Geometry check sheet. Reference: the model listing, model coordinates, mm. A direction names the side the tool comes from. Round coordinates to 2 decimals unless told otherwise and drop trailing zeros. Write each loop counter-clockwise with the first axis right and the second up, starting at its lowest first coordinate (ties: lowest second). Pieces come first, ordered by that corner, then holes. Notation, with made-up numbers: M 28,17 L 84,17 A15 cw 84,29 Z; hole C -5.75,59.5 d11. An arc over 180 degrees is marked long. Answer in a Markdown table with one row per item. Add a question column.
Autodesk Inventor part; units mm, degrees
ref_plane "YZ Plane" through (0, 0, 0) normal (1, 0, 0) x (0, 1, 0)
ref_plane "XZ Plane" through (0, 0, 0) normal (0, 1, 0) x (-1, 0, 0)
ref_plane "XY Plane" through (0, 0, 0) normal (0, 0, 1) x (1, 0, 0)
sketch "Sketch1" plane through (0, 0, 0) normal (0, 0, 1) x (1, 0, 0)
  line L0 (0, 0) -> (-18, 0)
  line L1 (-18, 0) -> (-19.55, 1.55)
  line L2 (-19.55, 1.55) -> (-19.55, 4.95)
  line L3 (-19.55, 4.95) -> (-18, 6.5)
  line L4 (-18, 6.5) -> (-14.45, 6.5)
  line L5 (-14.45, 6.5) -> (-14.45, 3.05)
  line L6 (-14.45, 3.05) -> (0, 3.05)
  line L7 (0, 3.05) -> (0, 0)
  point P0 (-19.55, 3.25)
  dimension "d0" = 3.05
  dimension "d1" = 14.45
  dimension "d2" = 6.5
  dimension "d3" = 5.1
  dimension "d4" = 3.4
  dimension "d5" = 3.25
  dimension "d6" = 3.55
extrude "Extrusion1" add sketch "Sketch1" along normal blind 0.55
ref_plane "Work Plane1" through (-14.45, 1.525, 0) normal (0, 1, 0) x (1, 0, 0)
sketch "Sketch2" plane through (-14.45, 1.525, 0) normal (0, 1, 0) x (1, 0, 0)
  line L0 (14.45, -0.55) -> (0, -0.55)
  line L1 (14.45, 0) -> (14.45, -0.55)
  line L2 (7.75, -0.55) -> (11.15, -0.55)
  line L3 (11.15, -0.55) -> (11.15, -2.25)
  line L4 (11.15, -2.25) -> (7.75, -2.25)
  line L5 (7.75, -2.25) -> (7.75, -0.55)
  line L6 (11.15, -0.55) -> (12.475, -1.875)
  line L7 (12.475, -1.875) -> (12.275, -0.55)
  line L8 (7.75, -0.55) -> (6.425, -1.875)
  line L9 (6.425, -1.875) -> (6.625, -0.55)
  line L10 (6.625, -0.55) -> (7.75, -0.55)
  line L11 (11.15, -0.55) -> (12.275, -0.55)
  point P0 (9.45, -2.25)
  dimension "d9" = 3.3
  dimension "d10" = 3.4
  dimension "d11" = 1.7
  dimension "d14" = 6.05
  dimension "d15" = 3.025
  dimension "d16" = 5.65
extrude "Extrusion2" add sketch "Sketch2" along normal mid plane 0.5
fillet "Fillet1" radius 0.2 2 edges at (-8.025, 1.525, 1.875) (-1.975, 1.525, 1.875)
properties part number "Soanar Power Module Pin E" material "Nickel-Copper Alloy 400"
Item 1: Section check D-D, the plane z = 1.8. Record the boundary of the cut face in (x, y) (3 decimals), and give its area (3 significant figures).
Item 2: Mould release check, pull along X, two halves, no side actions. Record for faces 1 (the flat face through (-2.86, 1.52, 0.99)), 2 (the flat face through (-18.8, 0.8, 0.3)), 3 (the flat face through (-2.6, 1.275, 0.9)): +X half, -X half, draft (parallel to the pull), parting line (faces both ways), or undercut.
Item 3: Section check A-A, the plane x = -6. Record the boundary of the cut face in (y, z) (3 decimals).
Item 4: Gauge pin test, flat ends, axial feed: pin 1 Ø0.5 at (x, z) = (-7, 1) entering from +Y (3 decimals); pin 2 Ø3.5 at (x, y) = (-14, 2.5) entering from +Z; pin 3 Ø0.8 at (x, z) = (-7.5, 1) entering from -Y (3 decimals). Record the tip position at first contact, or that the pin passes through.
Item 5: Access from +Z, -Z, +X, -X, +Y, -Y to the whole of each face (thin tool, end or side, straight path). Record for faces 4 (the flat face through (-18.8, 5.7, 0.3)), 5 (the flat face through (-12, 2, 0)), 6 (the flat face through (-7.5, 1.775, 0.9)), 7 (the flat face through (-7.14, 1.52, 0.99)), 8 (the flat face through (-5, 1.275, 1)).
Item 6: Section check C-C, the plane y = 4.5. Record the boundary of the cut face in (x, z), and give its area (4 significant figures).
Item 7: Section check B-B, the plane z = 1.05. Record the boundary of the cut face in (x, y) (3 decimals).
Item 8: Scan lines: probe 1 along Y at (x, z) = (-3.75, 0.7) (3 decimals); probe 2 along Y at (x, z) = (-2.25, 0.25); probe 3 along Z at (x, y) = (-4, 2.25). Record each from-to range of solid material in increasing order. Write a range as from..to.
Result sheet:
| question | item | result |
|---|---|---|
| 1 | outline | M -6.7,1.275 L -3.3,1.275 L -3.3,1.775 L -6.7,1.775 Z |
| 1 | area | 1.70 mm^2 |
| 2 | face 1 | undercut |
| 2 | face 2 | -X half |
| 2 | face 3 | draft |
| 3 | outline | M 0,0 L 3.05,0 L 3.05,0.55 L 1.775,0.55 L 1.775,2.25 L 1.275,2.25 L 1.275,0.55 L 0,0.55 Z |
| 4 | pin 1 | stops at y = 1.775 |
| 4 | pin 2 | stops at z = 0.55 |
| 4 | pin 3 | stops at y = 1.275 |
| 5 | face 4 | +Z, -Z, -X, +Y |
| 5 | face 5 | -Z, +X, -X, +Y, -Y |
| 5 | face 6 | +Z, +X, -X, +Y |
| 5 | face 7 | +Z, +Y, -Y |
| 5 | face 8 | +Z, +X, -X, -Y |
| 6 | outline | M -19.55,0 L -14.45,0 L -14.45,0.55 L -19.55,0.55 Z |
| 6 | area | 2.805 mm^2 |
| 7 | outline | M -7.9,1.275 L -7.2,1.275 L -7.2,1.775 L -7.9,1.775 Z; M -6.7,1.275 L -3.3,1.275 L -3.3,1.775 L -6.7,1.775 Z; M -2.8,1.275 L -2.1,1.275 L -2.1,1.775 L -2.8,1.775 Z |
| 8 | probe 1 | y = 1.275..1.775 |
| 8 | probe 2 | y = 0..3.05 |
| 8 | probe 3 | z = 0..0.55 |
